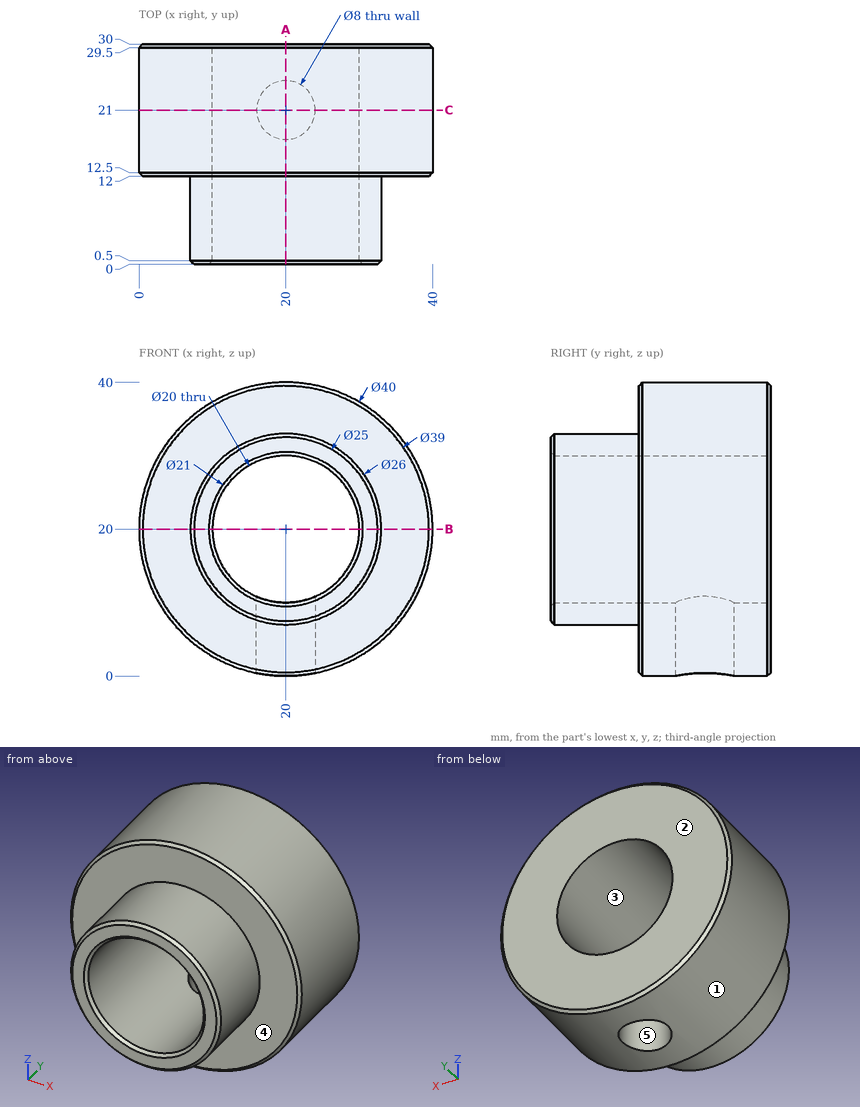
Answer from the drawing. Dimensions are ordinates in mm from the lowest x, y and z of the part. A direction names the side the tool comes from. Give positions to 0.01 mm unless a question says otherwise; leave off trailing zeros. Order: outer loops, then holes, each group sorted by start corner. A loop starts at its lowest first (then second) coordinate and runs counter-clockwise, first axis right, second up. Notation, with made-up numbers: (-8.5, -6) - (-0.5, -6) arc R18 cw to (-0.5, 8) - close; hole circle Ø3 at (73.5, 23.5). An arc over 180 degrees is marked (long way). One line per item, written item: value. Start each with the question number.
1. Section C-C, the plane y = 21 is taken. Write down the section's boundary in (x, z), then the cut area to 3 significant figures.
2. Section B-B, the plane z = 20 is taken. Write down the section's boundary in (x, y).
3. Section A-A, the plane x = 20 is taken. Write down the section's boundary in (y, z).
4. Each of these flat-tipped pins is pushed along its axis until it touches: pin 1 Ø1.5 at (x, z) = (15, 28) entering from +Y; pin 2 Ø6 at (x, y) = (22, 25.5) entering from +Z; pin 3 Ø10 at (x, y) = (24.5, 9) entering from -Z; pin 4 Ø6 at (y, z) = (12, 8.5) entering from +X. Where does it stop, or does it pass through?
5. Consider line 1 (Y direction, x = 20, z = 4); line 2 (Z direction, x = 20, y = 7); line 3 (Y direction, x = 6, z = 32). Determine where each line is inside the solid, lowest interval first.
6. For a pull along X with two mould halves and no side action, classify the marked faces 1, 2 and 3 as released by +X, released by -X, zero draft, split by the parting line, or undercut.
7. Which of the six approach directions +Z, -Z, +X, -X, +Y, -Y give full straight-line access (tool end or side, diameter ignored) to the marked faces 4 and 5?
Filled sheet:
1. outline: (16, 0.4) - (16, 10.83) arc R10 cw (long way) to (24, 10.83) - (24, 0.4) arc R20 ccw (long way) to start
1. area: 861 mm²
2. outline: (0, 12.5) - (0.5, 12) - (7, 12) - (7, 0.5) - (7.5, 0) - (9.5, 0) - (10, 0.5) - (10, 30) - (0.5, 30) - (0, 29.5) - close; (30, 0.5) - (30.5, 0) - (32.5, 0) - (33, 0.5) - (33, 12) - (39.5, 12) - (40, 12.5) - (40, 29.5) - (39.5, 30) - (30, 30) - close
3. outline: (0, 7.5) - (0.5, 7) - (12, 7) - (12, 0.5) - (12.5, 0) - (17, 0) - (17, 10) - (0.5, 10) - (0, 9.5) - close; (0, 30.5) - (0.5, 30) - (30, 30) - (30, 39.5) - (29.5, 40) - (12.5, 40) - (12, 39.5) - (12, 33) - (0.5, 33) - (0, 32.5) - close; (25, 0) - (29.5, 0) - (30, 0.5) - (30, 10) - (25, 10) - close
4. pin 1: y = 30
4. pin 2: z = 40
4. pin 3: z = 0.02
4. pin 4: x = 38.08
5. line 1: 12 to 17, 25 to 30
5. line 2: 7 to 10, 30 to 33
5. line 3: 12 to 30
6. face 1: split by the parting line
6. face 2: zero draft
6. face 3: undercut
7. face 4: -Y
7. face 5: -Z
